Model file for the job. Use its own axes, mm. Face numbers are marked on the shaded views. A direction names the side the tool comes from. Round coordinates to 2 decimals unless told otherwise and drop trailing zeros. Order: outer loops, then holes, each group sorted by start corner. A loop starts at its lowest first (then second) coordinate and runs counter-clockwise, first axis right, second up. Notation, with made-up numbers: (68, -5) - (112, -5) arc R31 ccw to (112, 23) - close; hole circle Ø10 at (82, -11). An arc over 180 degrees is marked (long way). Write item = value, one per line.
```python
from build123d import *

# Parameters (mm, degrees)
BOSS_EXTRUDE1_DEPTH = 70
SKETCH2_R           = 1.8
CUT_EXTRUDE1_DEPTH  = 262.101512826
CUT_EXTRUDE2_REACH  = 263.102


with BuildPart() as part:
    # Sketch1 → Boss-Extrude1 (new body)
    with BuildSketch(Plane(origin=(0, 0, 0), x_dir=(1, 0, 0), z_dir=(0, 1, 0))):
        Polygon((0, 0), (18, 0), (18, 57), (227, 57), (227, 0), (245, 0), (245, 3), (230, 3), (230, 60), (15, 60), (15, 3), (0, 3), align=None)
    extrude(amount=BOSS_EXTRUDE1_DEPTH)

    # Sketch2 → Cut-Extrude1 (cut, through all)
    with BuildSketch(Plane(origin=(0, 0, -3), x_dir=(-1, 0, 0), z_dir=(0, 0, -1))):
        with Locations((-240.02, 55)):
            Circle(SKETCH2_R)
        with Locations((-240.02, 35)):
            Circle(SKETCH2_R)
        with Locations((-240.02, 15)):
            Circle(SKETCH2_R)
        with Locations((-4.98, 15)):
            Circle(SKETCH2_R)
        with Locations((-4.98, 35)):
            Circle(SKETCH2_R)
        with Locations((-4.98, 55)):
            Circle(SKETCH2_R)
    extrude(amount=-CUT_EXTRUDE1_DEPTH, mode=Mode.SUBTRACT)

    # Sketch3 → Cut-Extrude2 (cut, up to next)
    with BuildSketch(Plane.XY.offset(-57), mode=Mode.PRIVATE) as cut_extrude2_sk1:
        with BuildLine():
            Line((110, 52.616114621), (110, 18.63325521))
            ThreePointArc((110, 18.63325521), (100, 8.63325521), (90, 18.63325521))
            Line((90, 18.63325521), (90, 52.616114621))
            ThreePointArc((90, 52.616114621), (100, 62.616114621), (110, 52.616114621))
        make_face()
    cut_extrude2_tool1 = extrude(cut_extrude2_sk1.sketch, amount=-CUT_EXTRUDE2_REACH, mode=Mode.PRIVATE) & part.part
    add(cut_extrude2_tool1.solids().sort_by_distance((100, 35.624685, -57))[0], mode=Mode.SUBTRACT)


solid = part.part
```
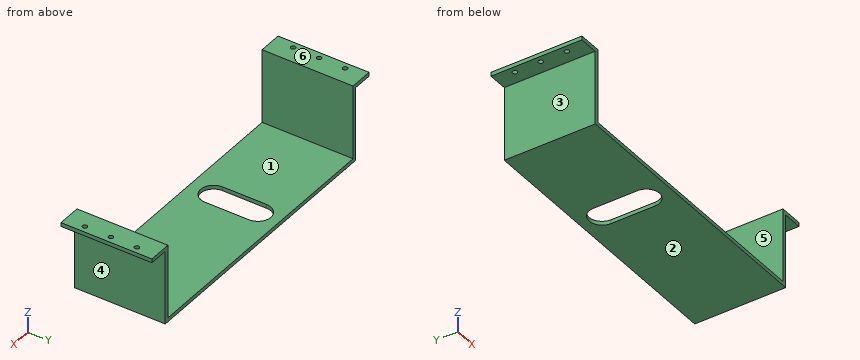
1) Mould opens along X. For the marked faces 4, 5 and 6 say: +X half, -X half, draft (parallel to the pull), parting line (faces both ways), or undercut.
Conclusion:
face_4 = +X half
face_5 = undercut
face_6 = draft
2) Cut at B-B (x = 100). Write the cut outline in (y, z), and give its area (3 significant figures).
Conclusion:
outline = (0, -60) - (8.63, -60) - (8.63, -57) - (0, -57) - close; (62.62, -60) - (70, -60) - (70, -57) - (62.62, -57) - close
area = 48.1 mm^2
3) Flat gauge pins, fed straight in: pin 1 Ø2 at (y, z) = (25, -8) entering from +X; pin 2 Ø12 at (x, y) = (4, 30.5) entering from -Z; pin 3 Ø1.5 at (y, z) = (46, -7) entering from -X; pin 4 Ø3 at (x, y) = (4.98, 35) entering from +Z. Where does each tip first touch, or does it go through?
Conclusion:
pin_1 = 230
pin_2 = -3
pin_3 = 15
pin_4 = through
4) Cut at A-A (y = 25). Write the cut outline in (x, z), and give its area (3 significant figures).
Conclusion:
outline = (0, -3) - (15, -3) - (15, -60) - (90, -60) - (90, -57) - (18, -57) - (18, 0) - (0, 0) - close; (110, -60) - (230, -60) - (230, -3) - (245, -3) - (245, 0) - (227, 0) - (227, -57) - (110, -57) - close
area = 1,020 mm^2
5) 3-axis set-ups, long thin cutter, end or side, ignore diameter. For the marked faces 1, 2 and 3: which of +Z, -Z, +X, -X, +Y, -Y reach the whole face in a straight line?
Conclusion:
face_1 = +Z, +Y, -Y
face_2 = -Z, +X, -X, +Y, -Y
face_3 = -Z, -X, +Y, -Y
6) Cut at D-D (x = 210). Write the cut outline in (y, z), and give its area (3 significant figures).
Conclusion:
outline = (0, -60) - (70, -60) - (70, -57) - (0, -57) - close
area = 210 mm^2
7) Wall check: line 1 along Y through (x, z) = (4.98, -1.6); line 2 along X through (y, z) = (24, -23); line 3 along Y through (x, z) = (4, -1). Give the ranges that are in metal, low to high.
Conclusion:
line_1 = 0 to 13.2, 16.8 to 33.2, 36.8 to 53.2, 56.8 to 70
line_2 = 15 to 18, 227 to 230
line_3 = 0 to 13.49, 16.51 to 33.49, 36.51 to 53.49, 56.51 to 70
8) Cut at C-C (z = -13). Write the cut outline in (x, y).
Conclusion:
outline = (15, 0) - (18, 0) - (18, 70) - (15, 70) - close; (227, 0) - (230, 0) - (230, 70) - (227, 70) - close
